from build123d import *

# Parameters (mm, degrees)
F1_DEPTH = 6.858
F2_R     = 4.57199
F3_R     = 6.35


# Not quite as in the source:
# - a fillet or chamfer is up to 0.001 mm smaller than in the source, because OpenCascade refuses the exact size


with BuildPart() as f1:
    # F0 (on Top) → F1 (new body)
    with BuildSketch(Plane.XY):
        Polygon((-7.62, -8.255), (7.62, -8.255), (7.62, 8.255), (4.572, 8.255), (4.572, -5.6657525711), (-4.572, -5.6657525711), (-4.572, 8.255), (-7.62, 8.255), align=None)
    extrude(amount=F1_DEPTH)

    # F2 (radius 4.572 in the source; OpenCascade refuses exactly that, so slightly less here)
    f2_edges = [f1.edges().sort_by_distance(p)[0] for p in [
        (-4.572, -5.665753, 3.429),
        (4.572, -5.665753, 3.429),
    ]]
    fillet(f2_edges, radius=F2_R)

    # F3
    f3_edges = [f1.edges().sort_by_distance(p)[0] for p in [
        (7.62, -8.255, 3.429),
        (-7.62, -8.255, 3.429),
    ]]
    fillet(f3_edges, radius=F3_R)


solid = f1.part
Geometry: final body of the model. Coordinates: model frame, mm. A direction names the side the tool comes from. Round coordinates to 2 decimals unless told otherwise and drop trailing zeros. Order: outer loops, then holes, each group sorted by start corner. A loop starts at its lowest first (then second) coordinate and runs counter-clockwise, first axis right, second up. Notation, with made-up numbers: (-31, 19.25) -> (22, 19.25) arc R14 cw to (22, 29.25) -> close; hole circle Ø1 at (31.25, -35). An arc over 180 degrees is marked (long way). Put each result on its own line as item: value. Start each with the question number.
Q1. First-contact query: pin 1 (2 mm diameter, centred on x = 1, z = 5, fed in from +Y); pin 2 (1.5 mm diameter, centred on y = -4, z = 4.5, fed in from -X). Flat tips, straight axial feed; report the tip coordinate or a pass-through.
Q2. Reachability of faces 1 (the flat face through (7.62, 3, 3)), 2 (the flat face through (-4.572, 4, 3)) from +Z, -Z, +X, -X, +Y, -Y: full face, straight path, thin tool, end or side. Return the list, or none.
Q3. Line query: probe 1 along X at (y, z) = (5.25, 3); probe 2 along X at (y, z) = (-3.75, 3.5); probe 3 along Y at (x, z) = (3.25, 1.25). Output: solid intervals per line, ascending.
Q4. Section A-A on y = 0. Return the cut outline in (x, z), and give its area (3 significant figures).
Q5. Section D-D on x = 5.5. Return the cut outline in (y, z) (3 decimals), and give its area (3 significant figures).
Q6. Section C-C on y = -2.25. Return the cut outline in (x, z).
Ans:
1. pin 1: stops at y = -5.21
1. pin 2: stops at x = -7.48
2. face 1: +Z, -Z, +X, +Y, -Y
2. face 2: +Z, -Z, +Y
3. probe 1: x = -7.62 to -4.57, 4.57 to 7.62
3. probe 2: x = -7.35 to -3.72, 3.72 to 7.35
3. probe 3: y = -7.94 to -4.31
4. outline: (-7.62, 0) -> (-4.57, 0) -> (-4.57, 6.86) -> (-7.62, 6.86) -> close; (4.57, 0) -> (7.62, 0) -> (7.62, 6.86) -> (4.57, 6.86) -> close
4. area: 41.8 mm2
5. outline: (-6.641, 0) -> (8.255, 0) -> (8.255, 6.858) -> (-6.641, 6.858) -> close
5. area: 102 mm2
6. outline: (-7.61, 0) -> (-4.42, 0) -> (-4.42, 6.86) -> (-7.61, 6.86) -> close; (4.42, 0) -> (7.61, 0) -> (7.61, 6.86) -> (4.42, 6.86) -> close
